Verification items for the finished model (mm, model axes). Face numbers are marked on the shaded views. Round coordinates to 2 decimals unless told otherwise and drop trailing zeros. Order: outer loops, then holes, each group sorted by start corner. A loop starts at its lowest first (then second) coordinate and runs counter-clockwise, first axis right, second up. Notation, with made-up numbers: (77, 50) -> (96, 50) arc R27 ccw to (96, 89) -> close; hole circle Ø6 at (53.5, 19). An arc over 180 degrees is marked (long way). Return JSON: item names as keys, results as strings. Group by question number.
1) Draft check along Z on the marked faces 1, 2, 3 and 4. Enter one of: pulls with the +Z half, pulls with the -Z half, needs draft (parallel to the pull), parting line crosses it, or undercut.
2) Section check C-C on z = 8.5. Enter the section's corners in (x, y), plus the area to 3 significant figures.
3) Depth check by flat-ended pin: pin 1 (5 mm diameter, centred on y = -3.5, z = 12, fed in from -X); pin 2 (6 mm diameter, centred on y = 1.5, z = 8.5, fed in from +X); pin 3 (1.5 mm diameter, centred on x = 8, z = 3, fed in from -Y). Enter the tip coordinate at first touch or a pass-through.
4) Section check A-A on x = 0. Enter the section's corners in (y, z), plus the area to 3 significant figures.
5) Scan lines: L1, parallel to Y at x = 0, z = 5.5; L2, parallel to Z at x = 9.75, y = 6.75; L3, parallel to X at y = 3.5, z = 13.5. Record each from-to range of solid material in increasing order.
```python
from build123d import *

# Parameters (mm, degrees)
SKETCH1_R           = 11.5
SKETCH1_R_2         = 9.5
BOSS_EXTRUDE1_DEPTH = 18.8
BOSS_EXTRUDE3_START = -0.5
SKETCH2_R           = 12.5
SKETCH2_R_2         = 11.5
BOSS_EXTRUDE3_DEPTH = 0.5
SKETCH3_R           = 12.5
SKETCH3_R_2         = 11.5
BOSS_EXTRUDE4_DEPTH = 0.5


with BuildPart() as part:
    # Sketch1 → Boss-Extrude1 (new body)
    with BuildSketch(Plane.XY):
        with Locations(Location((0, 0, 0), (0, 0, 180))):
            Circle(SKETCH1_R)
        with Locations(Location((0, 0, 0), (0, 0, 180))):
            Circle(SKETCH1_R_2, mode=Mode.SUBTRACT)
    extrude(amount=BOSS_EXTRUDE1_DEPTH)

    # Sketch2 → Boss-Extrude3 (add)
    with BuildSketch(Plane.XY.offset(18.8).offset(BOSS_EXTRUDE3_START)):
        Circle(SKETCH2_R)
        with Locations(Location((0, 0, 0), (0, 0, 180))):
            Circle(SKETCH2_R_2, mode=Mode.SUBTRACT)
    extrude(amount=BOSS_EXTRUDE3_DEPTH)

    # Sketch3 → Boss-Extrude4 (add)
    with BuildSketch(Plane(origin=(0, 0, 0), x_dir=(-1, 0, 0), z_dir=(0, 0, -1))):
        with Locations(Location((0, 0, 0), (0, 0, 180))):
            Circle(SKETCH3_R)
        Circle(SKETCH3_R_2, mode=Mode.SUBTRACT)
    extrude(amount=-BOSS_EXTRUDE4_DEPTH)


solid = part.part
```
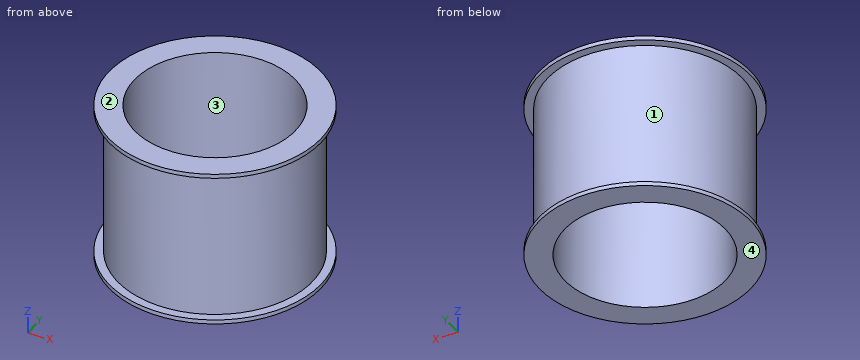
Check result:
{
 "1": {"face 1": "undercut", "face 2": "pulls with the +Z half", "face 3": "needs draft", "face 4": "pulls with the -Z half"},
 "2": {"outline": "circle Ø23 at (0, 0); hole circle Ø19 at (0, 0)", "area": "132 mm^2"},
 "3": {"pin 1": "x = -11.46", "pin 2": "x = 11.5", "pin 3": "y = -8.93"},
 "4": {"outline": "(-12.5, 0) -> (-9.5, 0) -> (-9.5, 18.8) -> (-12.5, 18.8) -> (-12.5, 18.3) -> (-11.5, 18.3) -> (-11.5, 0.5) -> (-12.5, 0.5) -> close; (9.5, 0) -> (12.5, 0) -> (12.5, 0.5) -> (11.5, 0.5) -> (11.5, 18.3) -> (12.5, 18.3) -> (12.5, 18.8) -> (9.5, 18.8) -> close", "area": "77.2 mm^2"},
 "5": {"L1": "-11.5 to -9.5, 9.5 to 11.5", "L2": "0 to 0.5, 18.3 to 18.8", "L3": "-10.95 to -8.83, 8.83 to 10.95"}
}
